from build123d import *

# Parameters (mm, degrees)
F1_DEPTH = 11.4
F3_R     = 3.6
F2_R     = 3.75


with BuildPart() as f1:
    # F0 (on Front) → F1 (new body, symmetric)
    with BuildSketch(Plane.XZ):
        Polygon((-1.262916, -6.812125), (5.268015, -4.49978), (6.530931, 2.312345), (1.262916, 6.812125), (-5.268015, 4.49978), (-6.530931, -2.312345), align=None)
    extrude(amount=F1_DEPTH, both=True)

    # F3 (on face) → F4 section 0
    with BuildSketch(Plane.XZ.offset(11.4)):
        Circle(F3_R)
    # F2 (on face) → F4 section 1
    with BuildSketch(Plane(origin=(0, 11.4, 0), x_dir=(-1, 0, 0), z_dir=(0, 1, 0))):
        Circle(F2_R)
    loft(mode=Mode.SUBTRACT)


solid = f1.part
The listing builds one solid part. Answer for the finished solid, in the listing's coordinates (mm). A direction names the side the tool comes from. Coordinates: 2 decimals unless noted, no trailing zeros. Order: outer loops, then holes, each group sorted by start corner. A loop starts at its lowest first (then second) coordinate and runs counter-clockwise, first axis right, second up.
Q1. Given P1, Ø5, axis at x = 1.5, z = 1, coming from the -Y side; P2, Ø4, axis at x = 3, y = -1.5, coming from the -Z side; P3, Ø2, axis at x = 3, y = 1.5, coming from the -Z side; P4, Ø2, axis at x = 4.5, y = -6, coming from the -Z side, each flat-ended and moving along its own axis, determine where each tip first touches the part or whether it passes through.
Q2. Which of the six approach directions +Z, -Z, +X, -X, +Y, -Y give full straight-line access (tool end or side, diameter ignored) to faces 1 (the face through (-0.479, 0.16, 3.645)), 2 (the face through (3, -11.4, -3))?
Q3. A cutting plane is placed at B-B, the plane x = -4. Write down the section's boundary in (y, z).
Q4. A cutting plane is placed at A-A, the plane z = -5. Write down the section's boundary in (x, y).
Q5. Consider line 1 (Z direction, x = -3, y = 3.5); line 2 (X direction, y = 1, z = -3); line 3 (X direction, y = -0.5, z = -1.25). Determine where each line is inside the solid, lowest interval first.
Answers follow:
1. P1: stops at y = -11.4
1. P2: stops at z = -6.01
1. P3: stops at z = -5.66
1. P4: stops at z = -5.13
2. face 1: +Y
2. face 2: +Z, -Z, +X, -X, -Y
3. outline: (-11.4, -4.47) - (11.4, -4.47) - (11.4, 4.95) - (-11.4, 4.95) - close
4. outline: (-3.38, -11.4) - (3.86, -11.4) - (3.86, 11.4) - (-3.38, 11.4) - close
5. line 1: z = -5.33 to -2.16, 2.16 to 5.3
5. line 2: x = -5.73 to -2.13, 2.13 to 5.55
5. line 3: x = -6.33 to -3.45, 3.45 to 5.87
